Here's how the part is built. I have some questions about the finished solid (model axes, mm). Coordinates: 2 decimals unless noted, no trailing zeros. Loops run counter-clockwise (first coordinate to the right, second up) from the corner with the lowest first, then second, coordinate; pieces in that order, holes last. Notation, with made-up numbers: (34, -27.5) -> (56, -27.5) arc R20 cw to (56, -6.5) -> close; hole circle Ø11 at (18, 36.5). An arc over 180 degrees is marked (long way). Answer as a JSON object with one key per item and string values. Group by question number.
Q1. I want a section at C-C on y = 8.5. Write out the boundary of the cut face in (x, z).
Q2. I want a section at B-B on y = 6. Write out the boundary of the cut face in (x, z), then the cut area to 3 significant figures.
Q3. I want a section at D-D on x = 8.25. Write out the boundary of the cut face in (y, z).
Q4. I want a section at A-A on y = -0.75. Write out the boundary of the cut face in (x, z).
Q5. I'm going to push flat-ended pins straight in: pin 1 (1 mm diameter, centred on y = -1.5, z = 1.5, fed in from -X); pin 2 (1 mm diameter, centred on y = 5, z = 1, fed in from +X); pin 3 (1.5 mm diameter, centred on y = -5, z = 1.5, fed in from -X); pin 4 (12 mm diameter, centred on x = 7, y = -4.5, fed in from -Z). Where does each tip first touch, or does it pass through?
Q6. I need wall thicknesses on line 1 (Y direction, x = 2, z = 0.8); line 2 (X direction, y = 7, z = 2.65); line 3 (X direction, y = 5, z = 0.7). Which ranges of each line are inside material? Lowest first, please.
```python
from build123d import *

# Parameters (mm, degrees)
F0_R            = 10
F0_R_2          = 7.6
F1_DEPTH        = 3
F3_DEPTH        = 3
F3_COPIES_COUNT = 15


# Not quite as in the source:
# - a pattern or mirror of a feature is missing from the dataset's text; its kind, count and spacing are read off the source's solid
# - a feature names something its author has since deleted; it is built from what else it names


with BuildPart() as f1:
    # F0 (on Top) → F1 (new body)
    with BuildSketch(Plane.XY):
        Circle(F0_R)
        Circle(F0_R_2, mode=Mode.SUBTRACT)
    extrude(amount=F1_DEPTH)

    # F2 (on Top) → F3 (join, through all)
    with BuildSketch(Plane.XY):
        with BuildLine():
            ThreePointArc((0, 3.9140510674), (-1.211569324, 6.0142199175), (0.6459488827, 7.57249959))
            ThreePointArc((0.6459488827, 7.57249959), (0, 7.6), (-0.6459488827, 7.57249959))
            ThreePointArc((-0.6459488827, 7.57249959), (-1.6403009124, 5.686249795), (-0.6459488827, 3.8))
            Line((-0.6459488827, 3.8), (0, 3.8))
            Line((0, 3.8), (0, 3.9140510674))
        make_face()
    f3 = extrude(amount=F3_DEPTH)

    # F3_copies: F3 ×15 about axis
    f3_copies_axis = Axis((0, 0, 0), (0, 0, 1))
    for i in range(1, F3_COPIES_COUNT):
        add(f3.rotate(f3_copies_axis, i * 360 / F3_COPIES_COUNT))


solid = f1.part
```
Result set:
{
 "1": {"outline": "(-5.27, 0) -> (5.27, 0) -> (5.27, 3) -> (-5.27, 3) -> close"},
 "2": {"outline": "(-8, 0) -> (-4.66, 0) -> (-4.66, 3) -> (-8, 3) -> close; (-3.94, 0) -> (-3.53, 0) -> (-3.53, 3) -> (-3.94, 3) -> close; (-1.62, 0) -> (-1.21, 0) -> (-1.21, 3) -> (-1.62, 3) -> close; (0.88, 0) -> (1.35, 0) -> (1.35, 3) -> (0.88, 3) -> close; (4.66, 0) -> (8, 0) -> (8, 3) -> (4.66, 3) -> close", "area": "23.9 mm²"},
 "3": {"outline": "(-5.65, 0) -> (5.65, 0) -> (5.65, 3) -> (-5.65, 3) -> close"},
 "4": {"outline": "(-9.97, 0) -> (-7.43, 0) -> (-7.43, 3) -> (-9.97, 3) -> close; (-4.01, 0) -> (-3.74, 0) -> (-3.74, 3) -> (-4.01, 3) -> close; (7.41, 0) -> (9.97, 0) -> (9.97, 3) -> (7.41, 3) -> close"},
 "5": {"pin 1": "stops at x = -9.95", "pin 2": "stops at x = 8.93", "pin 3": "stops at x = -9.05", "pin 4": "stops at z = 0"},
 "6": {"line 1": "y = -9.8 to -6.9, -4.49 to -3.93, 6.59 to 7.03, 7.33 to 9.8", "line 2": "x = -7.14 to -2.81, -1.23 to -0.71, 1.93 to 7.14", "line 3": "x = -8.66 to -5.54, -3.96 to -3.55, -1.53 to -1.11, 0.62 to 1.02, 3.1 to 3.79, 5.52 to 8.66"}
}
